Build history of the part. All positions in model axes, mm. A direction names the side the tool comes from. Round coordinates to 2 decimals unless told otherwise and drop trailing zeros. Write each loop counter-clockwise with the first axis right and the second up, starting at its lowest first coordinate (ties: lowest second). Pieces come first, ordered by that corner, then holes. Notation, with made-up numbers: M 63,70.5 L 82,70.5 A14 ccw 82,91.5 Z; hole C 18,2.25 d9. An arc over 180 degrees is marked long. Use a Markdown table: item, result.
from build123d import *

# Parameters (mm, degrees)
SZKIC1_R                    = 18
SZKIC1_R_2                  = 10.5
SZKIC1_R_3                  = 16
SZKIC1_R_4                  = 8
DODANIE_WYCI_GNI_CIE1_DEPTH = 7


with BuildPart() as part:
    # Szkic1 → Dodanie-wyciągnięcie1 (new body)
    # profile 1 of 3: a face of its own
    with BuildSketch(Plane.XY):
        with BuildLine():
            Line((68.906523061, 9), (29.071509826, 9))
            ThreePointArc((29.071509826, 9), (23.875357404, 12), (23.875357404, 18))
            Line((23.875357404, 18), (38.973056312, 44.149981587))
            ThreePointArc((38.973056312, 44.149981587), (39.641584345, 48.417073987), (37.271066361, 52.027565889))
            ThreePointArc((37.271066361, 52.027565889), (-37.146015536, 52.116921722), (-61.340613737, -18.257302823))
            ThreePointArc((-61.340613737, -18.257302823), (-58.51823129, -21.782574666), (-54.037016928, -22.341235641))
            Line((-54.037016928, -22.341235641), (-17.13928203, -12.454517373))
            ThreePointArc((-17.13928203, -12.454517373), (-14.262244941, -12.398004426), (-11.68977582, -13.687554248))
            ThreePointArc((-11.68977582, -13.687554248), (-17.112889149, -5.581131156), (-17.511771596, 4.163875068))
            ThreePointArc((-17.511771596, 4.163875068), (-19.046659036, 1.369774785), (-21.796114524, -0.243721533))
            Line((-21.796114524, -0.243721533), (-43.446394932, -6.044896685))
            ThreePointArc((-43.446394932, -6.044896685), (-48.638675969, -5.019562848), (-50.999217096, -0.282587291))
            ThreePointArc((-50.999217096, -0.282587291), (-29.136896009, 41.857392309), (17.972237006, 47.728384605))
            ThreePointArc((17.972237006, 47.728384605), (21.50727904, 44.134176714), (21.054008604, 39.113280534))
            Line((21.054008604, 39.113280534), (10.281653378, 20.455013964))
            ThreePointArc((10.281653378, 20.455013964), (7.514747752, 17.968780283), (3.814125716, 17.591260473))
            ThreePointArc((3.814125716, 17.591260473), (14.011678395, 11.299241946), (18, 0))
            ThreePointArc((18, 0), (16.984145827, -5.961441984), (14.051245496, -11.25))
            ThreePointArc((14.051245496, -11.25), (16.136917784, -9.591673087), (18.734993995, -9))
            Line((18.734993995, -9), (68.906523061, -9))
            ThreePointArc((68.906523061, -9), (71.299695166, -9.497934272), (73.295653135, -10.909090909))
            ThreePointArc((73.295653135, -10.909090909), (69, 0), (73.295653135, 10.909090909))
            ThreePointArc((73.295653135, 10.909090909), (71.299695166, 9.497934272), (68.906523061, 9))
        make_face()
    # profile 2 of 3: a face of its own
    with BuildSketch(Plane.XY):
        Circle(SZKIC1_R)
        Circle(SZKIC1_R_2, mode=Mode.SUBTRACT)
    # profile 3 of 3: a face of its own
    with BuildSketch(Plane.XY):
        with Locations((85, 0)):
            Circle(SZKIC1_R_3)
        with Locations((85, 0)):
            Circle(SZKIC1_R_4, mode=Mode.SUBTRACT)
    extrude(amount=DODANIE_WYCI_GNI_CIE1_DEPTH)


solid = part.part
Q1. Two-plate mould, pull along X, no slides. Class faces 1 (the cylindrical face through (-36.24, 52.75, 3.45)), 2 (the flat face through (-1, 12, 0)), 3 (the cylindrical face through (78.651, -4.868, 3.451)): +X half, -X half, draft (parallel to the pull), parting line (faces both ways), or undercut.
Response values:
| item | result |
|---|---|
| face 1 | parting line |
| face 2 | draft |
| face 3 | undercut |
Q2. Cut at C-C on z = 4.75. Count the separate pieces of the cut face and the enclosed holes in it, and give its area (3 significant figures).
Response values:
| item | result |
|---|---|
| separate pieces | 1 |
| enclosed holes | 3 |
| area | 5,150 mm2 |
Q3. Drill centre lines: L1, parallel to Y at x = 0, z = 1.5; L2, parallel to Y at x = 85, z = 3.25; L3, parallel to X at y = 2, z = 4.5. Where is each one in solid material? Low to high.
Response values:
| item | result |
|---|---|
| L1 | y = -18 to -10.5, 10.5 to 18, 51 to 64 |
| L2 | y = -16 to -8, 8 to 16 |
| L3 | x = -63.97 to -50.96, -18.51 to -10.31, 10.31 to 77.25, 92.75 to 100.87 |
Q4. Cut at B-B on x = 0. Give the cut face in (y, z), and give its area (3 significant figures).
Response values:
| item | result |
|---|---|
| outline | M -18,0 L -10.5,0 L -10.5,7 L -18,7 Z; M 10.5,0 L 18,0 L 18,7 L 10.5,7 Z; M 51,0 L 64,0 L 64,7 L 51,7 Z |
| area | 196 mm2 |
Q5. Cut at A-A on x = 85. Give the cut face in (y, z).
Response values:
| item | result |
|---|---|
| outline | M -16,0 L -8,0 L -8,7 L -16,7 Z; M 8,0 L 16,0 L 16,7 L 8,7 Z |
Q6. Drop flat-ended pins along their axis: P1, Ø2, axis at y = -5.5, z = 4.5, coming from the -X side; P2, Ø3, axis at y = 50, z = 4, coming from the -X side; P3, Ø6, axis at x = 43.5, y = 46.5, coming from the -Z side. Give the stop position or say it passes through.
Response values:
| item | result |
|---|---|
| P1 | stops at x = -63.84 |
| P2 | stops at x = -41.76 |
| P3 | passes through |
Q7. Which spindle directions (+Z, -Z, +X, -X, +Y, -Y) get a long thin tool onto all of the face, cutting with end or side? Do faces 4 (the cylindrical face through (-9.42, 15.34, 3.45)), 5 (the flat face through (-35.85, -17.47, 3.45)), 6 (the flat face through (31.319, 30.892, 3.451)). Say none if no direction does.
Response values:
| item | result |
|---|---|
| face 4 | +Z, -Z |
| face 5 | +Z, -Z, -Y |
| face 6 | +Z, -Z, +X |
Q8. Cut at D-D on y = 6. Give the cut face in (x, z).
Response values:
| item | result |
|---|---|
| outline | M -63.72,0 L -50.65,0 L -50.65,7 L -63.72,7 Z; M -16.97,0 L -8.62,0 L -8.62,7 L -16.97,7 Z; M 8.62,0 L 79.71,0 L 79.71,7 L 8.62,7 Z; M 90.29,0 L 99.83,0 L 99.83,7 L 90.29,7 Z |
